Can you work these out from the model? Positions are in its coordinate system, mm. A direction names the side the tool comes from. Round coordinates to 2 decimals unless told otherwise and drop trailing zeros. Loops run counter-clockwise (first coordinate to the right, second up) from the corner with the lowest first, then second, coordinate; pieces in that order, holes last. Notation, with made-up numbers: (7, -27) -> (31, -27) arc R26 ccw to (31, 5) -> close; hole circle Ø10 at (72.25, 43.25). An arc over 180 degrees is marked (long way). Use a Markdown table: item, result.
from build123d import *

# Parameters (mm, degrees)
SKETCH_W     = 50
SKETCH_H     = 40
PAD_DEPTH    = 0.5
PAD001_DEPTH = 5


with BuildPart() as part:
    # Sketch → Pad (new body)
    with BuildSketch(Plane.XY):
        with Locations((25, 20)):
            Rectangle(SKETCH_W, SKETCH_H)
    extrude(amount=PAD_DEPTH)

    # Sketch001 (on Face6 of Pad) → Pad001 (join)
    with BuildSketch(Plane.XY.offset(0.5)):
        Polygon((30, 5.35), (30, 4), (20, 4), (20, 5.35), (25, 5.35), align=None)
        Polygon((35, 15.35), (35, 16.7), (25, 16.7), (15, 16.7), (15, 15.35), (25, 15.35), align=None)
        Polygon((40, 25.35), (40, 26.7), (25, 26.7), (10, 26.7), (10, 25.35), (25, 25.35), align=None)
        Polygon((5, 35.35), (45, 35.35), (45, 36.7), (25, 36.7), (5, 36.7), align=None)
    extrude(amount=PAD001_DEPTH)


solid = part.part
1. I want a section at A-A (z = 3.35). Please give me the cut outline in (x, y), plus the area to 3 significant figures.
Answer sheet:
| item | result |
|---|---|
| outline | (5, 35.35) -> (45, 35.35) -> (45, 36.7) -> (5, 36.7) -> close; (10, 25.35) -> (40, 25.35) -> (40, 26.7) -> (10, 26.7) -> close; (15, 15.35) -> (35, 15.35) -> (35, 16.7) -> (15, 16.7) -> close; (20, 4) -> (30, 4) -> (30, 5.35) -> (20, 5.35) -> close |
| area | 135 mm² |
2. I want a section at B-B (x = 31.5). Please give me the cut outline in (y, z).
Answer sheet:
| item | result |
|---|---|
| outline | (0, 0) -> (40, 0) -> (40, 0.5) -> (36.7, 0.5) -> (36.7, 5.5) -> (35.35, 5.5) -> (35.35, 0.5) -> (26.7, 0.5) -> (26.7, 5.5) -> (25.35, 5.5) -> (25.35, 0.5) -> (16.7, 0.5) -> (16.7, 5.5) -> (15.35, 5.5) -> (15.35, 0.5) -> (0, 0.5) -> close |
3. I need wall thicknesses on line 1 (Y direction, x = 23, z = 3); line 2 (Y direction, x = 36, z = 2.45); line 3 (Z direction, x = 18, y = 23). Which ranges of each line are inside material? Lowest first, please.
Answer sheet:
| item | result |
|---|---|
| line 1 | y = 4 to 5.35, 15.35 to 16.7, 25.35 to 26.7, 35.35 to 36.7 |
| line 2 | y = 25.35 to 26.7, 35.35 to 36.7 |
| line 3 | z = 0 to 0.5 |
4. I want a section at D-D (x = 13). Please give me the cut outline in (y, z), plus the area to 3 significant figures.
Answer sheet:
| item | result |
|---|---|
| outline | (0, 0) -> (40, 0) -> (40, 0.5) -> (36.7, 0.5) -> (36.7, 5.5) -> (35.35, 5.5) -> (35.35, 0.5) -> (26.7, 0.5) -> (26.7, 5.5) -> (25.35, 5.5) -> (25.35, 0.5) -> (0, 0.5) -> close |
| area | 33.5 mm² |
5. If we mould it in two halves opening along Y, with no side actions, what happens to faces 5 (the flat face through (25, 5.35, 3)), 6 (the flat face through (30, 5, 3)), 7 (the flat face through (25, 4, 3))? For each: +Y half, -Y half, draft (parallel to the pull), parting line (faces both ways), or undercut.
Answer sheet:
| item | result |
|---|---|
| face 5 | undercut |
| face 6 | draft |
| face 7 | -Y half |
6. Which directions (+Z, -Z, +X, -X, +Y, -Y) give clear straight access to the entire face, cutting with the end or side of a thin tool? Please do faces 1 (the flat face through (45, 36, 3)), 2 (the flat face through (10, 26, 3)), 3 (the flat face through (25, 26.7, 3)), 4 (the flat face through (35, 16, 3)).
Answer sheet:
| item | result |
|---|---|
| face 1 | +Z, +X, +Y, -Y |
| face 2 | +Z, -X, -Y |
| face 3 | +Z, +X, -X |
| face 4 | +Z, +X, -Y |
7. Will these pins go through, and if not, where does the flat tip stop? pin 1 Ø0.7 at (y, z) = (36, 2) entering from +X; pin 2 Ø0.7 at (y, z) = (26, 3) entering from -X; pin 3 Ø1 at (x, z) = (31, 1.5) entering from -Y.
Answer sheet:
| item | result |
|---|---|
| pin 1 | stops at x = 45 |
| pin 2 | stops at x = 10 |
| pin 3 | stops at y = 15.35 |
8. I want a section at C-C (y = 31). Please give me the cut outline in (x, z), plus the area to 3 significant figures.
Answer sheet:
| item | result |
|---|---|
| outline | (0, 0) -> (50, 0) -> (50, 0.5) -> (0, 0.5) -> close |
| area | 25.0 mm² |
